Part model, mm, in its own coordinate system. Coordinates: 2 decimals unless noted, no trailing zeros. Loops run counter-clockwise (first coordinate to the right, second up) from the corner with the lowest first, then second, coordinate; pieces in that order, holes last. Notation, with made-up numbers: M 56.5,51.5 L 110.5,51.5 A12 ccw 110.5,66.5 Z; hole C -28.75,-15 d1. An arc over 180 degrees is marked long. Answer as a JSON object with one key per item and string values. Group by question number.
1. Drop flat-ended pins along their axis: pin 1 Ø5.5 at (x, y) = (0, -7.34) entering from +Z (3 decimals); pin 2 Ø4 at (y, z) = (-9.5, 7.5) entering from +X; pin 3 Ø3.5 at (x, y) = (0, 7.34) entering from -Z (3 decimals). Give the stop position or say it passes through.
2. Saw through at B-B on y = -10. Write the cut outline in (x, z) (3 decimals).
3. Saw through at A-A on z = 1. Write the cut outline in (x, y).
4. Saw through at C-C on x = -5.5. Write the cut outline in (y, z) (3 decimals), then the cut area to 3 significant figures.
5. Drill centre lines: L1, parallel to Y at x = -2, z = 3.75; L2, parallel to Y at x = -0.25, z = 3; L3, parallel to X at y = -5.75, z = 5.75. Where is each one in solid material? Low to high.
from build123d import *

# Parameters (mm, degrees)
F1_DEPTH = 15.875


with BuildPart() as f1:
    # F0 (on Top) → F1 (new body)
    with BuildSketch(Plane.XY):
        with BuildLine():
            ThreePointArc((0, 5.04825), (1.620936, 5.719664), (2.29235, 7.3406))
            ThreePointArc((2.29235, 7.3406), (-1.620936, 8.961536), (0, 5.04825))
        make_face()
        with BuildLine():
            ThreePointArc((2.29235, -7.3406), (1.620936, -5.719664), (0, -5.04825))
            ThreePointArc((0, -5.04825), (-1.620936, -8.961536), (2.29235, -7.3406))
        make_face()
        with BuildLine():
            Line((1.5875, 12.7), (-1.5875, 12.7))
            ThreePointArc((-1.5875, 12.7), (-6.077628, 10.840128), (-7.9375, 6.35))
            Line((-7.9375, 6.35), (-7.9375, -6.35))
            ThreePointArc((-7.9375, -6.35), (-6.077628, -10.840128), (-1.5875, -12.7))
            Line((-1.5875, -12.7), (1.5875, -12.7))
            ThreePointArc((1.5875, -12.7), (6.077628, -10.840128), (7.9375, -6.35))
            Line((7.9375, -6.35), (7.9375, 6.35))
            ThreePointArc((7.9375, 6.35), (6.077628, 10.840128), (1.5875, 12.7))
        make_face()
        with BuildLine():
            ThreePointArc((2.29235, -7.3406), (-1.620936, -8.961536), (0, -5.04825))
            ThreePointArc((0, -5.04825), (1.620936, -5.719664), (2.29235, -7.3406))
        make_face(mode=Mode.SUBTRACT)
        with BuildLine():
            ThreePointArc((0, 5.04825), (-1.620936, 8.961536), (2.29235, 7.3406))
            ThreePointArc((2.29235, 7.3406), (1.620936, 5.719664), (0, 5.04825))
        make_face(mode=Mode.SUBTRACT)
    extrude(amount=F1_DEPTH)


solid = f1.part
Outcome:
{
 "1": {"pin 1": "stops at z = 15.875", "pin 2": "stops at x = 7.83", "pin 3": "passes through"},
 "2": {"outline": "M -6.784,0 L 6.784,0 L 6.784,15.875 L -6.784,15.875 Z"},
 "3": {"outline": "M -7.94,-6.35 A6.35 ccw -1.59,-12.7 L 1.59,-12.7 A6.35 ccw 7.94,-6.35 L 7.94,6.35 A6.35 ccw 1.59,12.7 L -1.59,12.7 A6.35 ccw -7.94,6.35 Z; hole C 0,-7.34 d4.58; hole C 0,7.34 d4.58"},
 "4": {"outline": "M -11.351,0 L 11.351,0 L 11.351,15.875 L -11.351,15.875 Z", "area": "360 mm²"},
 "5": {"L1": "y = -12.69 to -8.46, -6.22 to 6.22, 8.46 to 12.69", "L2": "y = -12.7 to -9.62, -5.06 to 5.06, 9.62 to 12.7", "L3": "x = -7.94 to -1.65, 1.65 to 7.94"}
}
